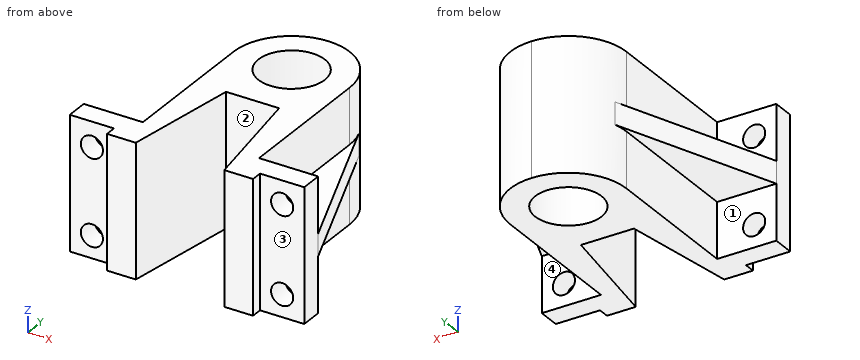
from build123d import *

# Parameters (mm, degrees)
BOSS_EXTRUDE1_DEPTH = 60
SKETCH3_R           = 15
CUT_EXTRUDE1_DEPTH  = 60
SKETCH4_R           = 5
CUT_EXTRUDE2_DEPTH  = 60
BOSS_EXTRUDE2_DEPTH = 5
BOSS_EXTRUDE3_DEPTH = 5


with BuildPart() as part:
    # Sketch2 → Boss-Extrude1 (new body)
    with BuildSketch(Plane.XY):
        with BuildLine():
            ThreePointArc((-1.497772579, 31.002473484), (-20.061398623, 23.31316781), (-27.750704297, 4.749541766))
            Line((-27.750704297, 4.749541766), (-1.497772579, 4.749541766))
            Line((-1.497772579, 4.749541766), (-1.497772579, 31.002473484))
        make_face()
        with BuildLine():
            Line((-1.497772579, 4.749541766), (-27.750704297, 4.749541766))
            ThreePointArc((-27.750704297, 4.749541766), (-20.061398623, -13.814084278), (-1.497772579, -21.503389952))
            Line((-1.497772579, -21.503389952), (-1.497772579, 4.749541766))
        make_face()
        with BuildLine():
            Line((24.75515914, 4.749541766), (-1.497772579, 4.749541766))
            Line((-1.497772579, 4.749541766), (-1.497772579, -21.503389952))
            ThreePointArc((-1.497772579, -21.503389952), (17.065853465, -13.814084278), (24.75515914, 4.749541766))
        make_face()
        with BuildLine():
            Line((-1.497772579, 31.002473484), (-1.497772579, 4.749541766))
            Line((-1.497772579, 4.749541766), (24.75515914, 4.749541766))
            ThreePointArc((24.75515914, 4.749541766), (17.065853465, 23.31316781), (-1.497772579, 31.002473484))
        make_face()
        with BuildLine():
            ThreePointArc((-1.497772579, -21.503389952), (-20.061398623, -13.814084278), (-27.750704297, 4.749541766))
            Line((-27.750704297, 4.749541766), (-27.750704297, -60.250458234))
            Line((-27.750704297, -60.250458234), (-54.497772579, -60.250458234))
            Line((-54.497772579, -60.250458234), (-54.497772579, -70.250458234))
            Line((-54.497772579, -70.250458234), (-34.497772579, -70.250458234))
            Line((-34.497772579, -70.250458234), (-34.497772579, -75.250458234))
            Line((-34.497772579, -75.250458234), (-21.497772579, -75.250458234))
            Line((-21.497772579, -75.250458234), (-13.497772579, -23.250458234))
            Line((-13.497772579, -23.250458234), (10.502227421, -23.250458234))
            Line((10.502227421, -23.250458234), (18.502227421, -75.250458234))
            Line((18.502227421, -75.250458234), (31.502227421, -75.250458234))
            Line((31.502227421, -75.250458234), (31.502227421, -70.250458234))
            Line((31.502227421, -70.250458234), (51.502227421, -70.250458234))
            Line((51.502227421, -70.250458234), (51.502227421, -60.250458234))
            Line((51.502227421, -60.250458234), (24.75515914, -60.250458234))
            Line((24.75515914, -60.250458234), (24.75515914, 4.749541766))
            ThreePointArc((24.75515914, 4.749541766), (17.065853465, -13.814084278), (-1.497772579, -21.503389952))
        make_face()
    extrude(amount=-BOSS_EXTRUDE1_DEPTH)

    # Sketch3 → Cut-Extrude1 (cut)
    with BuildSketch(Plane.XY):
        with Locations((-1.497772579, 4.749541766)):
            Circle(SKETCH3_R)
    extrude(amount=-CUT_EXTRUDE1_DEPTH, mode=Mode.SUBTRACT)

    # Sketch4 → Cut-Extrude2 (cut)
    with BuildSketch(Plane(origin=(0, -60.250458234, 0), x_dir=(1, 0, 0), z_dir=(0, 1, 0))):
        with Locations(Location((41.502227421, 10.524161434, 0), (0, 0, 270))):
            Circle(SKETCH4_R)
        with Locations(Location((41.502227421, 50, 0), (0, 0, 270))):
            Circle(SKETCH4_R)
        with Locations(Location((-44.497772579, 50, 0), (0, 0, 270))):
            Circle(SKETCH4_R)
        with Locations(Location((-44.497772579, 11.209528187, 0), (0, 0, 270))):
            Circle(SKETCH4_R)
    extrude(amount=-CUT_EXTRUDE2_DEPTH, mode=Mode.SUBTRACT)


with BuildPart() as part_1:
    # Body-Move/Copy1: moved
    add(part.part.moved(Location((0, 0, 30))))

    # Sketch5 → Boss-Extrude2 (add, symmetric)
    with BuildSketch(Plane.XY):
        Polygon((23.019364547, 14.137108595), (51.502227421, -60.250458234), (24.75515914, -60.250458234), (23.019364547, -60.250458234), align=None)
    extrude(amount=BOSS_EXTRUDE2_DEPTH, both=True)

    # Sketch7 → Boss-Extrude3 (add, symmetric)
    with BuildSketch(Plane.XY):
        Polygon((-54.497772579, -60.250458234), (-26.888977339, 11.420609494), (-26.888977339, -60.250458234), align=None)
    extrude(amount=BOSS_EXTRUDE3_DEPTH, both=True)


solid = part_1.part
Model file for the job. Use its own axes, mm. Face numbers are marked on the shaded views. A direction names the side the tool comes from. Give positions to 0.01 mm unless a question says otherwise; leave off trailing zeros. Loops run counter-clockwise (first coordinate to the right, second up) from the corner with the lowest first, then second, coordinate; pieces in that order, holes last. Notation, with made-up numbers: (71.25, 67.25) -> (98.25, 67.25) arc R29 cw to (98.25, 97.25) -> close; hole circle Ø3 at (-35, -15.75). An arc over 180 degrees is marked (long way). Use a Markdown table: item, result. Add a question column.
(1) Slice it at A-A on z = -20. List the corners of the cut face in (x, y).
(2) Slice it at B-B on z = -9.5. List the corners of the cut face in (x, y), and give its area (3 significant figures).
(3) Drop flat-ended pins along their axis: pin 1 Ø3 at (y, z) = (-2, -2) entering from -X; pin 2 Ø8 at (x, z) = (41.5, 19.48) entering from +Y; pin 3 Ø1.5 at (y, z) = (-73, -14.5) entering from +X; pin 4 Ø4 at (y, z) = (-4.5, 19.5) entering from -X. Give the stop position or say it passes through.
(4) Wall check: line 1 along X through (y, z) = (-67.5, -20); line 2 along X through (y, z) = (-66.75, -20); line 3 along Z through (x, y) = (-48.5, -65). Give the ranges that are in metal, low to high.
(5) Tool access for the marked faces 1, 2, 3 and 4: list every direction of +Z, -Z, +X, -X, +Y, -Y with a clear straight run to the whole face (end or side of a thin tool).
(6) Slice it at D-D on x = -3. List the corners of the cut face in (y, z).
(7) Slice it at C-C on y = -42. List the corners of the cut face in (x, z).
Filled sheet:
| question | item | result |
|---|---|---|
| 1 | outline | (-54.5, -70.25) -> (-49.5, -70.25) -> (-49.5, -60.25) -> (-54.5, -60.25) -> close; (-39.5, -70.25) -> (-34.5, -70.25) -> (-34.5, -75.25) -> (-21.5, -75.25) -> (-13.5, -23.25) -> (10.5, -23.25) -> (18.5, -75.25) -> (31.5, -75.25) -> (31.5, -70.25) -> (36.5, -70.25) -> (36.5, -60.25) -> (24.76, -60.25) -> (24.76, 4.75) arc R26.25 ccw to (-27.75, 4.75) -> (-27.75, -60.25) -> (-39.5, -60.25) -> close; (46.5, -70.25) -> (51.5, -70.25) -> (51.5, -60.25) -> (46.5, -60.25) -> close; hole circle Ø30 at (-1.5, 4.75) |
| 2 | outline | (-54.5, -70.25) -> (-34.5, -70.25) -> (-34.5, -75.25) -> (-21.5, -75.25) -> (-13.5, -23.25) -> (10.5, -23.25) -> (18.5, -75.25) -> (31.5, -75.25) -> (31.5, -70.25) -> (51.5, -70.25) -> (51.5, -60.25) -> (24.76, -60.25) -> (24.76, 4.75) arc R26.25 ccw to (-27.75, 4.75) -> (-27.75, -60.25) -> (-54.5, -60.25) -> close; hole circle Ø30 at (-1.5, 4.75) |
| 2 | area | 3,510 mm2 |
| 3 | pin 1 | x = -32.64 |
| 3 | pin 2 | through |
| 3 | pin 3 | x = 31.5 |
| 3 | pin 4 | x = -27.75 |
| 4 | line 1 | -54.5 to -49.5, -39.5 to -20.31, 17.31 to 36.5, 46.5 to 51.5 |
| 4 | line 2 | -54.5 to -49.5, -39.5 to -20.19, 17.19 to 36.5, 46.5 to 51.5 |
| 4 | line 3 | -30 to -23, -17 to 15.79, 21.79 to 30 |
| 5 | face 1 | -Z, -X, +Y |
| 5 | face 2 | +Z, -Z, -Y |
| 5 | face 3 | +Z, -Z, +X, -Y |
| 5 | face 4 | -Z, +X, +Y |
| 6 | outline | (-23.25, -30) -> (-10.18, -30) -> (-10.18, 30) -> (-23.25, 30) -> close; (19.67, -30) -> (30.96, -30) -> (30.96, 30) -> (19.67, 30) -> close |
| 7 | outline | (-47.47, -5) -> (-27.75, -5) -> (-27.75, -30) -> (-16.38, -30) -> (-16.38, 30) -> (-27.75, 30) -> (-27.75, 5) -> (-47.47, 5) -> close; (13.39, -30) -> (24.76, -30) -> (24.76, -5) -> (44.51, -5) -> (44.51, 5) -> (24.76, 5) -> (24.76, 30) -> (13.39, 30) -> close |
